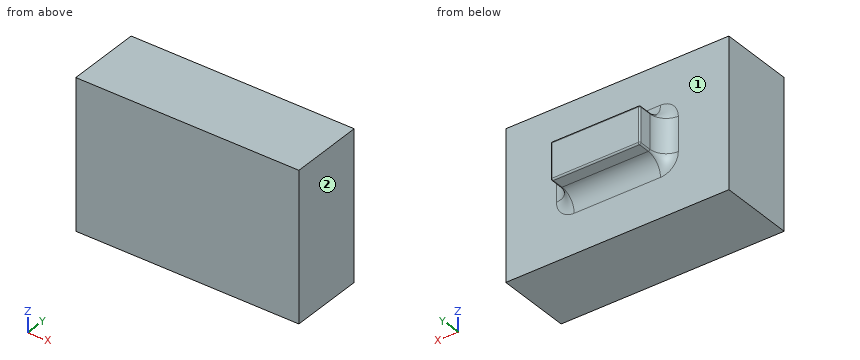
```python
from build123d import *

# Parameters (mm, degrees)
SKETCH_1_W      = 15
SKETCH_1_H      = 10
EXTRUDE_1_DEPTH = 5
SKETCH_2_W      = 6
SKETCH_2_H      = 2.5
EXTRUDE_2_DEPTH = 2
FILLET_1_R      = 0.1
FILLET_2_R      = 1.1
FILLET_3_R      = 0.1


with BuildPart() as part:
    # 草图1 → 凸台-拉伸1 (new body)
    with BuildSketch(Plane(origin=(0, 0, 0), x_dir=(1, 0, 0), z_dir=(0, 1, 0))):
        Rectangle(SKETCH_1_W, SKETCH_1_H)
    extrude(amount=EXTRUDE_1_DEPTH)

    # 草图2 → 凸台-拉伸2 (add)
    with BuildSketch(Plane(origin=(0, 5, 0), x_dir=(1, 0, 0), z_dir=(0, 1, 0))):
        Rectangle(SKETCH_2_W, SKETCH_2_H)
    extrude(amount=EXTRUDE_2_DEPTH)

    # 圆角1
    fillet_1_edges = [part.edges().sort_by_distance(p)[0] for p in [
        (-3, 6, -1.25),
        (-3, 6, 1.25),
        (3, 6, 1.25),
        (3, 6, -1.25),
    ]]
    fillet(fillet_1_edges, radius=FILLET_1_R)

    # 圆角2
    fillet_2_edges = [part.edges().sort_by_distance(p)[0] for p in [
        (-3, 5, 0),
        (0, 5, -1.25),
        (3, 5, 0),
        (0, 5, 1.25),
        (-2.970710678, 5, -1.220710678),
        (2.970710678, 5, -1.220710678),
        (2.970710678, 5, 1.220710678),
        (-2.970710678, 5, 1.220710678),
    ]]
    fillet(fillet_2_edges, radius=FILLET_2_R)

    # 圆角3
    fillet_3_edges = [part.edges().sort_by_distance(p)[0] for p in [
        (-3, 7, 0),
        (0, 7, -1.25),
        (0, 7, 1.25),
        (3, 7, 0),
        (-2.970710678, 7, 1.220710678),
        (2.970710678, 7, 1.220710678),
        (2.970710678, 7, -1.220710678),
        (-2.970710678, 7, -1.220710678),
    ]]
    fillet(fillet_3_edges, radius=FILLET_3_R)


solid = part.part
```
Could you check a few things on this model? Use its own coordinates, in mm. Face numbers are marked on the shaded views. A direction names the side the tool comes from. Give positions to 0.01 mm unless a question says otherwise; leave off trailing zeros. Order: outer loops, then holes, each group sorted by start corner. A loop starts at its lowest first (then second) coordinate and runs counter-clockwise, first axis right, second up.
Q1. Suppose I cut it at D-D, the plane z = -2.75. Write out the boundary of the cut face in (x, y), and give its area (3 significant figures).
Q2. If I drill on line 1 along Y through (x, z) = (5.25, 3); line 2 along Z through (x, y) = (-1.75, 6.5); line 3 along Y through (x, z) = (0, 1.75), over which ranges is the centre line in solid material (lowest first)?
Q3. Suppose I cut it at A-A, the plane z = 0.5. Write out the boundary of the cut face in (x, y), and give its area (3 significant figures).
Q4. Suppose I cut it at C-C, the plane y = 5.25. Write out the boundary of the cut face in (x, z).
Q5. I'm going to push flat-ended pins straight in: P1, Ø0.6, axis at x = -0.5, y = 6.5, coming from the +Z side; P2, Ø3, axis at x = -5.5, y = 6, coming from the +Z side. Where does each tip first touch, or does it pass through?
Q6. For the marked faces 1 and 2, which set-ups out of +Z, -Z, +X, -X, +Y, -Y let a thin tool reach every point of the face, with its end or its side?
Q7. Suppose I cut it at B-B, the plane x = -0.5. Write out the boundary of the cut face in (y, z), and give its area (3 significant figures).
Solution:
1. outline: (-7.5, 0) - (7.5, 0) - (7.5, 5) - (-7.5, 5) - close
1. area: 75.0 mm2
2. line 1: y = 0 to 5
2. line 2: z = -1.25 to 1.25
2. line 3: y = 0 to 5.18
3. outline: (-7.5, 0) - (7.5, 0) - (7.5, 5) - (4.1, 5) arc R1.1 cw to (3, 6.1) - (3, 6.9) arc R0.1 ccw to (2.9, 7) - (-2.9, 7) arc R0.1 ccw to (-3, 6.9) - (-3, 6.1) arc R1.1 cw to (-4.1, 5) - (-7.5, 5) - close
3. area: 87.5 mm2
4. outline: (-3.4, -1.15) arc R0.5 ccw to (-2.9, -1.65) - (2.9, -1.65) arc R0.5 ccw to (3.4, -1.15) - (3.4, 1.15) arc R0.5 ccw to (2.9, 1.65) - (-2.9, 1.65) arc R0.5 ccw to (-3.4, 1.15) - close
5. P1: stops at z = 1.25
5. P2: stops at z = 5
6. face 1: +Y
6. face 2: +Z, -Z, +X, +Y, -Y
7. outline: (0, -5) - (5, -5) - (5, -2.35) arc R1.1 cw to (6.1, -1.25) - (6.9, -1.25) arc R0.1 ccw to (7, -1.15) - (7, 1.15) arc R0.1 ccw to (6.9, 1.25) - (6.1, 1.25) arc R1.1 cw to (5, 2.35) - (5, 5) - (0, 5) - close
7. area: 55.5 mm2
